CAD build for the part. Positions are in the model's coordinates, mm. Give positions to 0.01 mm unless a question says otherwise; leave off trailing zeros. Loops run counter-clockwise (first coordinate to the right, second up) from the corner with the lowest first, then second, coordinate; pieces in that order, holes last.
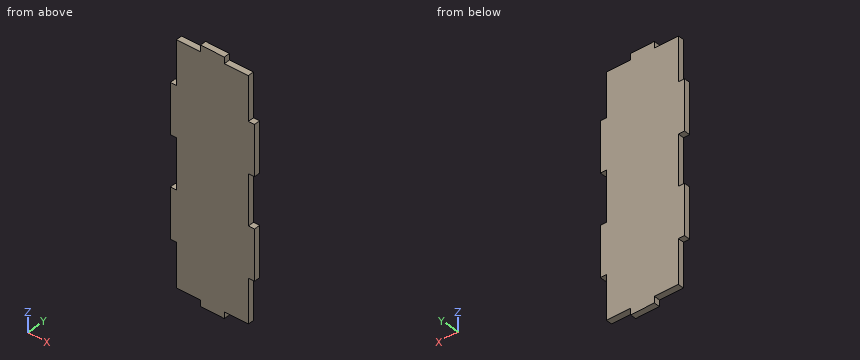
Autodesk Inventor part; units mm, degrees
ref_plane "YZ Plane" through (0, 0, 0) normal (1, 0, 0) x (0, 1, 0)
ref_plane "XZ Plane" through (0, 0, 0) normal (0, 1, 0) x (-1, 0, 0)
ref_plane "XY Plane" through (0, 0, 0) normal (0, 0, 1) x (1, 0, 0)
sketch "Sketch1" plane through (0, 0, 0) normal (0, 1, 0) x (-1, 0, 0)
  line L0 (-2.5, -54) -> (-2.5, -54)
  line L1 (-2.5, -54) -> (2.5, -54)
  line L2 (2.5, -54) -> (2.5, -54)
  line L3 (-12.5, -54) -> (-12.5, -54)
  line L4 (-12.5, -54) -> (-7.5, -54)
  line L5 (-7.5, -54) -> (-7.5, -54)
  line L6 (12.5, -54) -> (12.5, -54)
  line L7 (12.5, -54) -> (7.5, -54)
  line L8 (7.5, -54) -> (7.5, -54)
  line L9 (7.5, 60) -> (7.5, 60)
  line L10 (7.5, 60) -> (12.5, 60)
  line L11 (12.5, 60) -> (12.5, 60)
  line L12 (-2.5, 60) -> (-2.5, 60)
  line L13 (-2.5, 60) -> (2.5, 60)
  line L14 (2.5, 60) -> (2.5, 60)
  line L15 (-12.5, 60) -> (-12.5, 60)
  line L16 (-12.5, 60) -> (-7.5, 60)
  line L17 (-7.5, 60) -> (-7.5, 60)
  line L18 (17.5, 60) -> (17.5, 60)
  line L19 (17.5, -54) -> (17.5, -54)
  line L20 (-17.5, 60) -> (-17.5, 60)
  line L21 (-17.5, -54) -> (-17.5, -54)
  line L22 (17.5, -54) -> (17.5, -54)
  line L23 (17.5, 60) -> (17.5, 60)
  line L24 (12.5, -54) -> (17.5, -54)
  line L25 (2.5, -54) -> (7.5, -54)
  line L26 (-17.5, -54) -> (-12.5, -54)
  line L27 (-7.5, -54) -> (-2.5, -54)
  line L28 (-17.5, 60) -> (-17.5, 60)
  line L29 (-17.5, -54) -> (-17.5, -54)
  line L30 (-12.5, 60) -> (-17.5, 60)
  line L31 (-2.5, 60) -> (-7.5, 60)
  line L32 (17.5, 60) -> (12.5, 60)
  line L33 (7.5, 60) -> (2.5, 60)
  line L34 (17.5, -33) -> (20.5, -33)
  line L35 (20.5, -33) -> (20.5, -9)
  line L36 (20.5, -9) -> (17.5, -9)
  line L37 (17.5, 39) -> (20.5, 39)
  line L38 (20.5, 39) -> (20.5, 15)
  line L39 (20.5, 15) -> (17.5, 15)
  line L40 (-17.5, 39) -> (-20.5, 39)
  line L41 (-20.5, 39) -> (-20.5, 15)
  line L42 (-20.5, 15) -> (-17.5, 15)
  line L43 (-17.5, -9) -> (-20.5, -9)
  line L44 (-20.5, -9) -> (-20.5, -33)
  line L45 (-20.5, -33) -> (-17.5, -33)
  line L46 (17.5, -33) -> (17.5, -54)
  line L47 (17.5, 60) -> (17.5, 39)
  line L48 (17.5, 15) -> (17.5, -9)
  line L49 (-17.5, 60) -> (-17.5, 39)
  line L50 (-17.5, 15) -> (-17.5, -9)
  line L51 (-17.5, -33) -> (-17.5, -54)
  line L52 (5.8333, 60) -> (-5.8333, 60)
  line L53 (-5.8333, 60) -> (-5.8333, 63)
  line L54 (-5.8333, 63) -> (5.8333, 63)
  line L55 (5.8333, 63) -> (5.8333, 60)
  line L56 (5.8333, -54) -> (-5.8333, -54)
  line L57 (-5.8333, -54) -> (-5.8333, -57)
  line L58 (-5.8333, -57) -> (5.8333, -57)
  line L59 (5.8333, -57) -> (5.8333, -54)
  point P0 (0, 0)
  point P1 (-17.5, 50)
  point P2 (-17.5, -44)
  point P3 (17.5, -44)
  point P4 (17.5, 50)
  point P5 (-5.8333, 60)
  dimension "d40" = 35
  dimension "d49" = 0
  dimension "d50" = 0
  dimension "d55" = 17.5
  dimension "d56" = 60
  dimension "d57" = 114
  dimension "d58" = 0
  dimension "d59" = 0
  dimension "d62" = 24
  dimension "d63" = 24
  dimension "d65" = 3
  dimension "d66" = 21
  dimension "d67" = 11.6667
  dimension "d68" = 11.6667
  dimension "d69" = 3
  dimension "d70" = 3
extrude "Extrusion1" add sketch "Sketch1" along normal blind 3
equation "\"d40\" = shelfH"
equation "\"d57\" = -2 * tt + ht"
equation "\"d62\" = 0.2 * ht + 2 * tol"
equation "\"d63\" = 0.2 * ht - 2 * tol"
equation "\"d65\" = tt"
equation "\"d66\" = 0.2 * ht - tt"
equation "\"d67\" = 0.333333 * shelfH + 2 * tol"
equation "\"d68\" = 0.333333 * shelfH - tol"
equation "\"d69\" = tt"
equation "\"d70\" = tt"
equation "\"d31\" = tt"
equation "\"d4\" = tt"
equation "\"tt\" = 3"
equation "\"tol\" = 0"
equation "\"tiroir\" = 1"
equation "\"nHoles\" = 4"
equation "\"shelfH\" = 35"
equation "\"d42\" = 0.5 * shelfH"
equation "\"d43\" = 0.5 * shelfH"
properties part number "base"
1. Probe line 1 along Z through (x, y) = (-14, 0.3); line 2 along X through (y, z) = (0.35, 8). List the from-to ranges inside material, lowest first.
Responses:
line 1: z = -54 to 60
line 2: x = -17.5 to 17.5
2. Drop flat-ended pins along their axis: pin 1 (1.5 mm diameter, centred on y = 1.5, z = 53, fed in from +X); pin 2 (1.5 mm diameter, centred on y = 1, z = -44, fed in from -X); pin 3 (0.9 mm diameter, centred on x = 13.5, y = 1, fed in from -Z). Give the stop position or say it passes through.
Responses:
pin 1: stops at x = 17.5
pin 2: stops at x = -17.5
pin 3: stops at z = -54
3. Saw through at C-C, the plane z = -45. List the corners of the cut face in (x, y), and give its area (3 significant figures).
Responses:
outline: (-17.5, 0) - (17.5, 0) - (17.5, 3) - (-17.5, 3) - close
area: 105 mm2
4. Saw through at A-A, the plane y = 1.7. List the corners of the cut face in (x, z), and give its area (3 significant figures).
Responses:
outline: (-20.5, -33) - (-17.5, -33) - (-17.5, -54) - (-5.83, -54) - (-5.83, -57) - (5.83, -57) - (5.83, -54) - (17.5, -54) - (17.5, -33) - (20.5, -33) - (20.5, -9) - (17.5, -9) - (17.5, 15) - (20.5, 15) - (20.5, 39) - (17.5, 39) - (17.5, 60) - (5.83, 60) - (5.83, 63) - (-5.83, 63) - (-5.83, 60) - (-17.5, 60) - (-17.5, 39) - (-20.5, 39) - (-20.5, 15) - (-17.5, 15) - (-17.5, -9) - (-20.5, -9) - close
area: 4,350 mm2
5. Saw through at B-B, the plane x = -14. List the corners of the cut face in (y, z), and give its area (3 significant figures).
Responses:
outline: (0, -54) - (3, -54) - (3, 60) - (0, 60) - close
area: 342 mm2
